from build123d import *

# Parameters (mm, degrees)
SKETCH_7_R            = 1.65
EXTRUDE_542_DEPTH     = 2
SKETCH_8_R            = 2.75
CUT_EXTRUDE_611_DEPTH = 1.1


with BuildPart() as part:
    # 草图7 → Extrude 542 (new body)
    with BuildSketch(Plane.XY):
        Polygon((-60, -98), (60, -98), (72, -86), (72, 86), (60, 98), (-60, 98), (-72, 86), (-72, -86), align=None)
        with Locations((-20, -85)):
            Circle(SKETCH_7_R, mode=Mode.SUBTRACT)
        with Locations((-62, -28)):
            Circle(SKETCH_7_R, mode=Mode.SUBTRACT)
        with Locations((-28, -88)):
            Circle(SKETCH_7_R, mode=Mode.SUBTRACT)
        with Locations((-62, -40)):
            Circle(SKETCH_7_R, mode=Mode.SUBTRACT)
        with Locations((-20, 85)):
            Circle(SKETCH_7_R, mode=Mode.SUBTRACT)
        with Locations((-62, 28)):
            Circle(SKETCH_7_R, mode=Mode.SUBTRACT)
        with Locations((-28, 88)):
            Circle(SKETCH_7_R, mode=Mode.SUBTRACT)
        with Locations((-62, 40)):
            Circle(SKETCH_7_R, mode=Mode.SUBTRACT)
        with Locations((20, -85)):
            Circle(SKETCH_7_R, mode=Mode.SUBTRACT)
        with Locations((62, -28)):
            Circle(SKETCH_7_R, mode=Mode.SUBTRACT)
        with Locations((28, -88)):
            Circle(SKETCH_7_R, mode=Mode.SUBTRACT)
        with Locations((62, -40)):
            Circle(SKETCH_7_R, mode=Mode.SUBTRACT)
        with Locations((20, 85)):
            Circle(SKETCH_7_R, mode=Mode.SUBTRACT)
        with Locations((62, 28)):
            Circle(SKETCH_7_R, mode=Mode.SUBTRACT)
        with Locations((28, 88)):
            Circle(SKETCH_7_R, mode=Mode.SUBTRACT)
        with Locations((62, 40)):
            Circle(SKETCH_7_R, mode=Mode.SUBTRACT)
        with Locations((-46, -32.5)):
            Circle(SKETCH_7_R, mode=Mode.SUBTRACT)
        with Locations((-46, 46.5)):
            Circle(SKETCH_7_R, mode=Mode.SUBTRACT)
        with Locations((46, -32.5)):
            Circle(SKETCH_7_R, mode=Mode.SUBTRACT)
        with Locations((46, 46.5)):
            Circle(SKETCH_7_R, mode=Mode.SUBTRACT)
        Polygon((-64, -9), (-60, -9), (-58, -7), (-58, 7), (-60, 9), (-64, 9), (-66, 7), (-66, -7), align=None, mode=Mode.SUBTRACT)
        Polygon((-21, 56), (-13, 56), (-10, 59), (-10, 77), (-13, 80), (-21, 80), (-24, 77), (-24, 59), align=None, mode=Mode.SUBTRACT)
        Polygon((-21, -80), (-13, -80), (-10, -77), (-10, -59), (-13, -56), (-21, -56), (-24, -59), (-24, -77), align=None, mode=Mode.SUBTRACT)
        Polygon((60, -9), (64, -9), (66, -7), (66, 7), (64, 9), (60, 9), (58, 7), (58, -7), align=None, mode=Mode.SUBTRACT)
        Polygon((13, 56), (21, 56), (24, 59), (24, 77), (21, 80), (13, 80), (10, 77), (10, 59), align=None, mode=Mode.SUBTRACT)
        Polygon((13, -80), (21, -80), (24, -77), (24, -59), (21, -56), (13, -56), (10, -59), (10, -77), align=None, mode=Mode.SUBTRACT)
        Polygon((-12, -16), (12, -16), (16, -12), (16, 12), (12, 16), (-12, 16), (-16, 12), (-16, -12), align=None, mode=Mode.SUBTRACT)
    extrude(amount=EXTRUDE_542_DEPTH)

    # 草图8 → Cut-Extrude 611 (cut)
    with BuildSketch(Plane.XY):
        with Locations((-46, -32.5)):
            Circle(SKETCH_8_R)
        with Locations((-46, 46.5)):
            Circle(SKETCH_8_R)
        with Locations((46, -32.5)):
            Circle(SKETCH_8_R)
        with Locations((46, 46.5)):
            Circle(SKETCH_8_R)
    extrude(amount=CUT_EXTRUDE_611_DEPTH, mode=Mode.SUBTRACT)


solid = part.part
Source: CAD feature listing. Evaluate the final solid. Frame: model axes, mm. A direction names the side the tool comes from. Round coordinates to 2 decimals unless told otherwise and drop trailing zeros. Order: outer loops, then holes, each group sorted by start corner. A loop starts at its lowest first (then second) coordinate and runs counter-clockwise, first axis right, second up. Notation, with made-up numbers: (-6, -5.5) - (43, -5.5) arc R15 cw to (43, 20.5) - close; hole circle Ø1 at (62.5, 62.25). An arc over 180 degrees is marked (long way). Use a Markdown table: item, result. Add a question column.
1. Set-up query: faces 4 (the flat face through (-14, -14, 1)), 5 (the flat face through (66, -92, 1)), 6 (the flat face through (-45, 45, 1.1)). Return all of +Z, -Z, +X, -X, +Y, -Y with unobstructed straight access to the full face (end or side cutting, diameter ignored); none if empty.
2. Line query: probe 1 along X at (y, z) = (72.5, 0.1); probe 2 along Y at (x, z) = (-18, 1.9); probe 3 along Y at (x, z) = (46, 0.8). Output: solid intervals per line, ascending.
3. Mould query, pull axis Y, two halves, no side actions, for faces 1 (the flat face through (-66, 92, 1)), 2 (the flat face through (-17, 1, 0)), 3 (the cylindrical face through (43.973, -30.641, 0.542)). Classes: +Y half, -Y half, draft (parallel to the pull), parting line (faces both ways), or undercut.
4. First-contact query: pin 1 (6 mm diameter, centred on x = 20.5, y = 56, fed in from -Z). Flat tip, straight axial feed; report the tip coordinate or a pass-through.
5. Section query A-A (y = 2). Return the cut outline in (x, z), then the cut area to 3 significant figures.
6. Section query C-C (z = 0.65). Give the number of separate pieces and of enclosed holes in the cut face, then the cut area to 3 significant figures.
7. Section query B-B (y = -63). Return the cut outline in (x, z).
Derived:
| question | item | result |
|---|---|---|
| 1 | face 4 | +Z, -Z |
| 1 | face 5 | +Z, -Z, +X, -Y |
| 1 | face 6 | -Z |
| 2 | probe 1 | -72 to -24, -10 to 10, 24 to 72 |
| 2 | probe 2 | -98 to -80, -56 to 56, 80 to 98 |
| 2 | probe 3 | -98 to -35.25, -29.75 to 43.75, 49.25 to 98 |
| 3 | face 1 | +Y half |
| 3 | face 2 | draft |
| 3 | face 3 | undercut |
| 4 | pin 1 | z = 0 |
| 5 | outline | (-72, 0) - (-66, 0) - (-66, 2) - (-72, 2) - close; (-58, 0) - (-16, 0) - (-16, 2) - (-58, 2) - close; (16, 0) - (58, 0) - (58, 2) - (16, 2) - close; (66, 0) - (72, 0) - (72, 2) - (66, 2) - close |
| 5 | area | 192 mm2 |
| 6 | separate pieces | 1 |
| 6 | enclosed holes | 27 |
| 6 | area | 25,200 mm2 |
| 7 | outline | (-72, 0) - (-24, 0) - (-24, 2) - (-72, 2) - close; (-10, 0) - (10, 0) - (10, 2) - (-10, 2) - close; (24, 0) - (72, 0) - (72, 2) - (24, 2) - close |
